Geometry check sheet. Reference: drawing and pictorial views, mm from the part's lowest x, y, z. A direction names the side the tool comes from. Give positions to 0.01 mm unless a question says otherwise; leave off trailing zeros. Write each loop counter-clockwise with the first axis right and the second up, starting at its lowest first coordinate (ties: lowest second). Pieces come first, ordered by that corner, then holes. Notation, with made-up numbers: (30, 60) -> (62, 60) arc R18 ccw to (62, 80) -> close; hole circle Ø9 at (-16, 87.25). An arc over 180 degrees is marked (long way). Use a Markdown table: item, result. Add a question column.
1. Cross-section at C-C (z = 1.25). Enter the section's corners in (x, y).
2. Release check for a two-part mould opening along Z. For the marked faces 1, 2 and 3 record: released by +Z, released by -Z, zero draft, split by the parting line, or undercut.
3. Cross-section at A-A (x = 7.5). Enter the section's corners in (y, z), then the cut area to 3 significant figures.
4. Set-up check for the marked faces 4 and 5: record each of +Z, -Z, +X, -X, +Y, -Y from which the full face is reachable in a straight line by a thin tool's end or side.
5. Gauge pin test, flat ends, axial feed: P1, Ø1.5, axis at y = 8.5, z = 3, coming from the +X side; P2, Ø3, axis at x = 12, z = 5.5, coming from the +Y side; P3, Ø3, axis at x = 7.5, y = 7.5, coming from the +Z side; P4, Ø4, axis at x = 12, z = 2, coming from the -Y side. Record the tip position at first contact, or that the pin passes through.
6. Cross-section at D-D (x = 13). Enter the section's corners in (y, z).
7. Scan lines: probe 1 along Y at (x, z) = (7.5, 6.75); probe 2 along Z at (x, y) = (1, 4.5); probe 3 along X at (y, z) = (6, 0.5). Record each from-to range of solid material in increasing order. Write a range as [from, to].
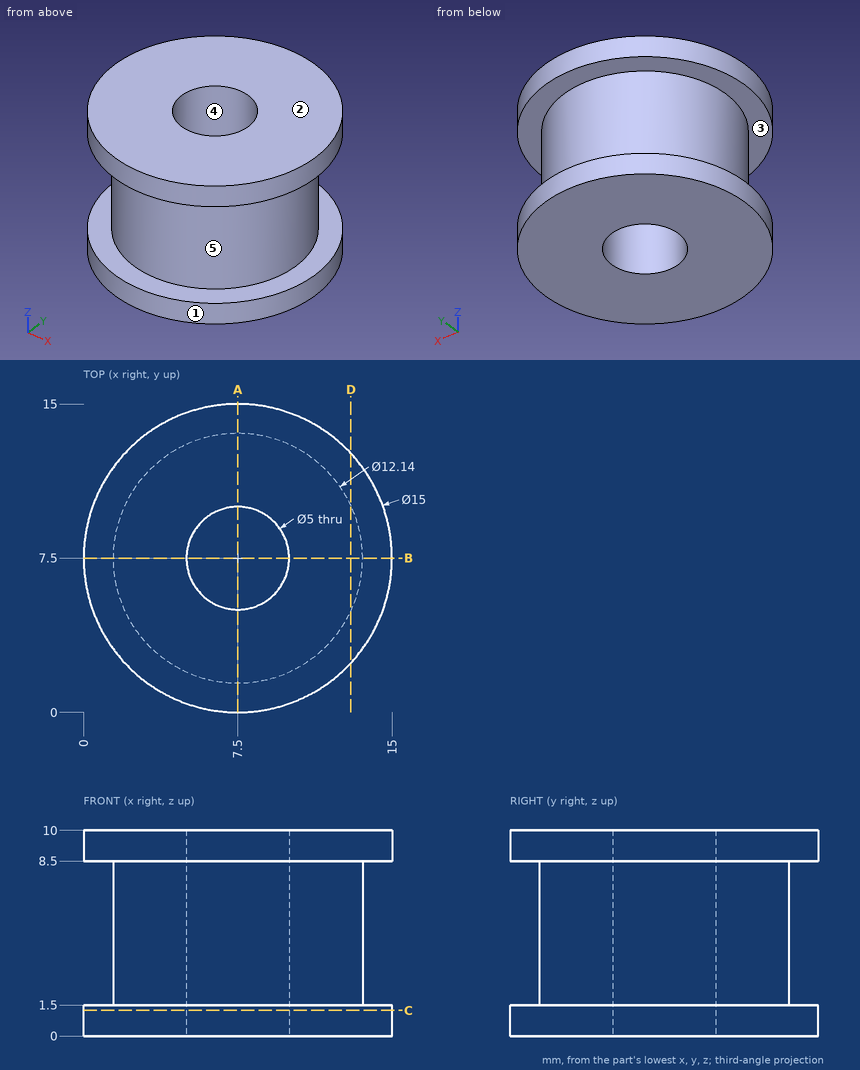
Worked answers:
| question | item | result |
|---|---|---|
| 1 | outline | circle Ø15 at (7.5, 7.5); hole circle Ø5 at (7.5, 7.5) |
| 2 | face 1 | zero draft |
| 2 | face 2 | released by +Z |
| 2 | face 3 | undercut |
| 3 | outline | (0, 0) -> (5, 0) -> (5, 10) -> (0, 10) -> (0, 8.5) -> (1.43, 8.5) -> (1.43, 1.5) -> (0, 1.5) -> close; (10, 0) -> (15, 0) -> (15, 1.5) -> (13.57, 1.5) -> (13.57, 8.5) -> (15, 8.5) -> (15, 10) -> (10, 10) -> close |
| 3 | area | 80.0 mm² |
| 4 | face 4 | +Z, -Z |
| 4 | face 5 | none |
| 5 | P1 | stops at x = 13.56 |
| 5 | P2 | stops at y = 12.78 |
| 5 | P3 | passes through |
| 5 | P4 | stops at y = 0.45 |
| 6 | outline | (2.4, 0) -> (12.6, 0) -> (12.6, 1.5) -> (10.07, 1.5) -> (10.07, 8.5) -> (12.6, 8.5) -> (12.6, 10) -> (2.4, 10) -> (2.4, 8.5) -> (4.93, 8.5) -> (4.93, 1.5) -> (2.4, 1.5) -> close |
| 7 | probe 1 | y = [1.43, 5], [10, 13.57] |
| 7 | probe 2 | z = [0, 1.5], [8.5, 10] |
| 7 | probe 3 | x = [0.15, 5.5], [9.5, 14.85] |
